```python
from build123d import *

# Parameters (mm, degrees)
SKETCH1_R           = 3.5
SKETCH1_R_2         = 0.1
SKETCH1_R_3         = 1.5
BOSS_EXTRUDE2_DEPTH = 10
SKETCH7_W           = 2.087565374
SKETCH7_H           = 50
BOSS_EXTRUDE4_DEPTH = 6


with BuildPart() as part:
    # Sketch1 → Boss-Extrude2 (new body)
    with BuildSketch(Plane(origin=(0, 0, 0), x_dir=(1, 0, 0), z_dir=(0, 1, 0))):
        with Locations(Location((0, 0, 0), (0, 0, 270))):
            Circle(SKETCH1_R)
        with Locations(Location((-1.606969024, 1.915111108, 0), (0, 0, 270))):
            Circle(SKETCH1_R_2, mode=Mode.SUBTRACT)
        with Locations(Location((-1.25, 2.165063509, 0), (0, 0, 270))):
            Circle(SKETCH1_R_2, mode=Mode.SUBTRACT)
        with Locations(Location((-0.855050358, 2.349231552, 0), (0, 0, 270))):
            Circle(SKETCH1_R_2, mode=Mode.SUBTRACT)
        with Locations(Location((-0.434120444, 2.462019383, 0), (0, 0, 270))):
            Circle(SKETCH1_R_2, mode=Mode.SUBTRACT)
        with Locations(Location((0, 2.5, 0), (0, 0, 270))):
            Circle(SKETCH1_R_2, mode=Mode.SUBTRACT)
        with Locations(Location((0.434120444, 2.462019383, 0), (0, 0, 270))):
            Circle(SKETCH1_R_2, mode=Mode.SUBTRACT)
        with Locations(Location((0.855050358, 2.349231552, 0), (0, 0, 270))):
            Circle(SKETCH1_R_2, mode=Mode.SUBTRACT)
        with Locations(Location((1.25, 2.165063509, 0), (0, 0, 270))):
            Circle(SKETCH1_R_2, mode=Mode.SUBTRACT)
        with Locations(Location((1.606969024, 1.915111108, 0), (0, 0, 270))):
            Circle(SKETCH1_R_2, mode=Mode.SUBTRACT)
        with Locations(Location((1.915111108, 1.606969024, 0), (0, 0, 270))):
            Circle(SKETCH1_R_2, mode=Mode.SUBTRACT)
        with Locations(Location((2.165063509, 1.25, 0), (0, 0, 270))):
            Circle(SKETCH1_R_2, mode=Mode.SUBTRACT)
        with Locations(Location((2.349231552, 0.855050358, 0), (0, 0, 270))):
            Circle(SKETCH1_R_2, mode=Mode.SUBTRACT)
        with Locations(Location((2.462019383, 0.434120444, 0), (0, 0, 270))):
            Circle(SKETCH1_R_2, mode=Mode.SUBTRACT)
        with Locations(Location((2.349231552, -0.855050358, 0), (0, 0, 270))):
            Circle(SKETCH1_R_2, mode=Mode.SUBTRACT)
        with Locations(Location((2.462019383, -0.434120444, 0), (0, 0, 270))):
            Circle(SKETCH1_R_2, mode=Mode.SUBTRACT)
        with Locations(Location((1.25, -2.165063509, 0), (0, 0, 270))):
            Circle(SKETCH1_R_2, mode=Mode.SUBTRACT)
        with Locations(Location((1.606969024, -1.915111108, 0), (0, 0, 270))):
            Circle(SKETCH1_R_2, mode=Mode.SUBTRACT)
        with Locations(Location((1.915111108, -1.606969024, 0), (0, 0, 270))):
            Circle(SKETCH1_R_2, mode=Mode.SUBTRACT)
        with Locations(Location((2.165063509, -1.25, 0), (0, 0, 270))):
            Circle(SKETCH1_R_2, mode=Mode.SUBTRACT)
        with Locations(Location((2.5, 0, 0), (0, 0, 270))):
            Circle(SKETCH1_R_2, mode=Mode.SUBTRACT)
        with Locations(Location((0.434120444, -2.462019383, 0), (0, 0, 270))):
            Circle(SKETCH1_R_2, mode=Mode.SUBTRACT)
        with Locations(Location((0.855050358, -2.349231552, 0), (0, 0, 270))):
            Circle(SKETCH1_R_2, mode=Mode.SUBTRACT)
        with Locations(Location((-0.434120444, -2.462019383, 0), (0, 0, 270))):
            Circle(SKETCH1_R_2, mode=Mode.SUBTRACT)
        with Locations(Location((-0.855050358, -2.349231552, 0), (0, 0, 270))):
            Circle(SKETCH1_R_2, mode=Mode.SUBTRACT)
        with Locations(Location((0, -2.5, 0), (0, 0, 270))):
            Circle(SKETCH1_R_2, mode=Mode.SUBTRACT)
        with Locations(Location((-1.25, -2.165063509, 0), (0, 0, 270))):
            Circle(SKETCH1_R_2, mode=Mode.SUBTRACT)
        with Locations(Location((-1.915111108, -1.606969024, 0), (0, 0, 270))):
            Circle(SKETCH1_R_2, mode=Mode.SUBTRACT)
        with Locations(Location((-1.606969024, -1.915111108, 0), (0, 0, 270))):
            Circle(SKETCH1_R_2, mode=Mode.SUBTRACT)
        with Locations(Location((-2.462019383, -0.434120444, 0), (0, 0, 270))):
            Circle(SKETCH1_R_2, mode=Mode.SUBTRACT)
        with Locations(Location((-2.349231552, -0.855050358, 0), (0, 0, 270))):
            Circle(SKETCH1_R_2, mode=Mode.SUBTRACT)
        with Locations(Location((-2.165063509, -1.25, 0), (0, 0, 270))):
            Circle(SKETCH1_R_2, mode=Mode.SUBTRACT)
        with Locations(Location((-2.349231552, 0.855050358, 0), (0, 0, 270))):
            Circle(SKETCH1_R_2, mode=Mode.SUBTRACT)
        with Locations(Location((-2.462019383, 0.434120444, 0), (0, 0, 270))):
            Circle(SKETCH1_R_2, mode=Mode.SUBTRACT)
        with Locations(Location((-2.5, 0, 0), (0, 0, 270))):
            Circle(SKETCH1_R_2, mode=Mode.SUBTRACT)
        with Locations(Location((-1.915111108, 1.606969024, 0), (0, 0, 270))):
            Circle(SKETCH1_R_2, mode=Mode.SUBTRACT)
        with Locations(Location((-2.165063509, 1.25, 0), (0, 0, 270))):
            Circle(SKETCH1_R_2, mode=Mode.SUBTRACT)
        with Locations(Location((0, 0, 0), (0, 0, 270))):
            Circle(SKETCH1_R_3, mode=Mode.SUBTRACT)
    extrude(amount=BOSS_EXTRUDE2_DEPTH)

    # Sketch7 → Boss-Extrude4 (add)
    with BuildSketch(Plane(origin=(0, 0, 0), x_dir=(1, 0, 0), z_dir=(0, 1, 0))):
        with Locations((0, -28.340736102)):
            Rectangle(SKETCH7_W, SKETCH7_H)
    extrude(amount=BOSS_EXTRUDE4_DEPTH)


solid = part.part
```
Geometry check sheet. Reference: the model listing, model coordinates, mm. A direction names the side the tool comes from. Coordinates: 2 decimals unless noted, no trailing zeros. Loops run counter-clockwise (first coordinate to the right, second up) from the corner with the lowest first, then second, coordinate; pieces in that order, holes last. Notation, with made-up numbers: (-25.75, 45.5) - (23.25, 45.5) arc R25 ccw to (23.25, 70.5) - close; hole circle Ø10 at (-35.75, 8). An arc over 180 degrees is marked (long way). One line per item, written item: value. Start each with the question number.
(1) Material ranges on line 1 (X direction, y = 4.5, z = 0); line 2 (Y direction, x = -1, z = 13); line 3 (X direction, y = 1, z = 12), recorded low to high. Write a range as [from, to].
(2) Cross-section at A-A on y = 7.5. Count the separate pieces of the cut face and the enclosed holes in it, plus the area to 3 significant figures.
(3) Depth check by flat-ended pin: P1, Ø1, axis at x = 2.5, z = 27, coming from the -Y side; P2, Ø5, axis at y = 2, z = 25, coming from the -X side; P3, Ø5, axis at y = 3, z = 9, coming from the +X side; P4, Ø4, axis at x = 1.5, y = 7, coming from the -Z side. Enter the tip coordinate at first touch or a pass-through.
(4) Mould release check, pull along Z, two halves, no side actions. Record for faces 4 (the cylindrical face through (0.45, 4.93, 1.43)), 5 (the flat face through (-1.044, 3, 29)), 6 (the cylindrical face through (-3.417, 4.93, -0.759)), 7 (the flat face through (0, 3, 53.341)): released by +Z, released by -Z, zero draft, split by the parting line, or undercut.
(5) Tool access check on faces 1 (the flat face through (1.044, 3, 29)), 2 (the flat face through (0, 6, 28)), 3 (the flat face through (0, 10, 2)). Record the directions out of +Z, -Z, +X, -X, +Y, -Y that give a thin tool (end or side, any length) a straight path to the whole face; none if there is none.
(6) Cross-section at B-B on z = 27.5. Enter the section's corners in (x, y), plus the area to 3 significant figures.
Results below:
1. line 1: x = [-3.5, -2.6], [-2.4, -1.5], [1.5, 2.4], [2.6, 3.5]
1. line 2: y = [0, 6]
1. line 3: x = [-1.04, 1.04]
2. separate pieces: 1
2. enclosed holes: 37
2. area: 30.3 mm2
3. P1: passes through
3. P2: stops at x = -1.04
3. P3: stops at x = 1.04
3. P4: stops at z = -3.5
4. face 4: undercut
4. face 5: zero draft
4. face 6: split by the parting line
4. face 7: released by +Z
5. face 1: +Z, +X, +Y, -Y
5. face 2: +Z, +X, -X, +Y
5. face 3: +Z, -Z, +X, -X, +Y
6. outline: (-1.04, 0) - (1.04, 0) - (1.04, 6) - (-1.04, 6) - close
6. area: 12.5 mm2
